```python
from build123d import *

# Parameters (mm, degrees)
SKETCH1_R           = 7.5
SKETCH1_R_2         = 5
BOSS_EXTRUDE1_DEPTH = 5
SKETCH2_R           = 6.5
BOSS_EXTRUDE2_DEPTH = 19
SKETCH4_W           = 21.748753338
SKETCH4_H           = 30.770097212
SKETCH4_W_2         = 12
SKETCH4_H_2         = 21.36247908
CUT_EXTRUDE1_DEPTH  = 38
SKETCH5_R           = 5
CUT_EXTRUDE2_DEPTH  = 5
SKETCH6_R           = 5
CUT_EXTRUDE3_DEPTH  = 37


with BuildPart() as part:
    # Sketch1 → Boss-Extrude1 (new body)
    with BuildSketch(Plane.XY):
        Circle(SKETCH1_R)
        Circle(SKETCH1_R_2, mode=Mode.SUBTRACT)
    extrude(amount=BOSS_EXTRUDE1_DEPTH)

    # Sketch2 → Boss-Extrude2 (add)
    with BuildSketch(Plane(origin=(0, 0, 0), x_dir=(-1, 0, 0), z_dir=(0, 0, -1))):
        Circle(SKETCH2_R)
    extrude(amount=BOSS_EXTRUDE2_DEPTH)

    # Sketch3 → Revolve9 (revolve)
    with BuildSketch(Plane(origin=(0, 0, 0), x_dir=(1, 0, 0), z_dir=(0, 1, 0))):
        with BuildLine():
            Line((0, 29), (0, 9))
            ThreePointArc((0, 9), (-10, 19), (0, 29))
        make_face()
    revolve(axis=Axis((0, 0, -29), (0, 0, 1)))

    # Sketch4 → Cut-Extrude1 (cut)
    with BuildSketch(Plane.XY.offset(5)):
        Rectangle(SKETCH4_W, SKETCH4_H)
        Rectangle(SKETCH4_W_2, SKETCH4_H_2, mode=Mode.SUBTRACT)
    extrude(amount=-CUT_EXTRUDE1_DEPTH, mode=Mode.SUBTRACT)

    # Sketch5 → Cut-Extrude2 (cut)
    with BuildSketch(Plane.XY):
        Circle(SKETCH5_R)
    extrude(amount=-CUT_EXTRUDE2_DEPTH, mode=Mode.SUBTRACT)

    # Sketch6 → Cut-Extrude3 (cut)
    with BuildSketch(Plane(origin=(6, 0, 0), x_dir=(0, 0, -1), z_dir=(1, 0, 0))):
        with Locations((19, 0)):
            Circle(SKETCH6_R)
    extrude(amount=-CUT_EXTRUDE3_DEPTH, mode=Mode.SUBTRACT)


solid = part.part
```
Geometry check sheet. Reference: the model listing, model coordinates, mm. A direction names the side the tool comes from. Coordinates: 2 decimals unless noted, no trailing zeros. Order: outer loops, then holes, each group sorted by start corner. A loop starts at its lowest first (then second) coordinate and runs counter-clockwise, first axis right, second up.
Item 1: Mould release check, pull along Y, two halves, no side actions. Record for faces 4 (the flat face through (-6, 0, -11)), 5 (the cylindrical face through (0.1, 7.5, 2.5)), 6 (the cylindrical face through (0, 0, -14)): released by +Y, released by -Y, zero draft, split by the parting line, or undercut.
Item 2: Section check A-A (z = -19). Enter the section's corners in (x, y).
Item 3: Section check B-B (x = 0). Enter the section's corners in (y, z), plus the area to 3 significant figures.
Item 4: Depth check by flat-ended pin: pin 1 (5 mm diameter, centred on y = -7, z = -2.5, fed in from -X); pin 2 (1.5 mm diameter, centred on x = -2.5, z = -11, fed in from +Y); pin 3 (6 mm diameter, centred on x = -4.5, z = -5, fed in from +Y); pin 4 (8 mm diameter, centred on y = -5, z = -11, fed in from -X). Enter the tip coordinate at first touch or a pass-through.
Item 5: Section check D-D (z = 2). Enter the section's corners in (x, y), plus the area to 3 significant figures.
Item 6: Section check C-C (y = -1.25). Enter the section's corners in (x, z), plus the area to 3 significant figures.
Item 7: Tool access check on faces 1 (the cylindrical face through (-0.1, -7.5, 2.5)), 2 (the flat face through (0, 7, 0)), 3 (the flat face through (0, 0, -5)). Record the directions out of +Z, -Z, +X, -X, +Y, -Y that give a thin tool (end or side, any length) a straight path to the whole face; none if there is none.
Item 8: Scan lines: line 1 along Y through (x, z) = (0, -0.25); line 2 along Y through (x, z) = (4.5, -20.5); line 3 along Z through (x, y) = (-3.75, 1.5). Record each from-to range of solid material in increasing order.
Check sheet entries:
1. face 4: zero draft
1. face 5: released by +Y
1. face 6: undercut
2. outline: (-6, -8) arc R10 ccw to (6, -8) - (6, -5) - (-6, -5) - close; (-6, 5) - (6, 5) - (6, 8) arc R10 ccw to (-6, 8) - close
3. outline: (-7.5, 0) - (-6.5, 0) - (-6.5, -11.4) arc R10 ccw (long way) to (6.5, -11.4) - (6.5, 0) - (7.5, 0) - (7.5, 5) - (5, 5) - (5, -5) - (-5, -5) - (-5, 5) - (-7.5, 5) - close; hole circle Ø10 at (0, -19)
3. area: 337 mm2
4. pin 1: stops at x = -4.69
4. pin 2: stops at y = 6.46
4. pin 3: stops at y = 6.32
4. pin 4: stops at x = -6
5. outline: (-6, -4.5) arc R7.5 ccw to (6, -4.5) - (6, 4.5) arc R7.5 ccw to (-6, 4.5) - close; hole circle Ø10 at (0, 0)
5. area: 79.8 mm2
6. outline: (-6, -26.9) arc R9.92 ccw to (6, -26.9) - (6, -23.84) - (-6, -23.84) - close; (-6, -14.16) - (6, -14.16) - (6, 5) - (4.84, 5) - (4.84, -5) - (-4.84, -5) - (-4.84, 5) - (-6, 5) - close
6. area: 186 mm2
7. face 1: +Z, -Y
7. face 2: +Y
7. face 3: +Z
8. line 1: y = -6.5 to -5, 5 to 6.5
8. line 2: y = -8.8 to -4.77, 4.77 to 8.8
8. line 3: z = -28.15 to -23.77, -14.23 to -5
